from build123d import *

# Parameters (mm, degrees)
SKETCH_1_R          = 1.7
EXTRUDE_1_DEPTH     = 39
FILLET_1_R          = 10
SKETCH_3_R          = 1.7
EXTRUDE_2_DEPTH     = 5
EXTRUDE_START       = -3
SKETCH_4_R          = 1.7
EXTRUDE_3_DEPTH     = 3
CUT_EXTRUDE_2_DEPTH = 5
SKETCH_6_R          = 1.7
EXTRUDE_4_DEPTH     = 3
SKETCH_7_R          = 1.7
EXTRUDE_5_DEPTH     = 5
SKETCH_8_R          = 3
SKETCH_8_R_2        = 1.7
EXTRUDE_6_DEPTH     = 39
SKETCH_9_R          = 1.7
CUT_EXTRUDE_3_DEPTH = 100
FILLET_2_R          = 10


with BuildPart() as part:
    # 草图1 → 凸台-拉伸1 (new body)
    with BuildSketch(Plane(origin=(0, 0, 0), x_dir=(1, 0, 0), z_dir=(0, 1, 0))):
        with BuildLine():
            Line((-14.277701198, -3), (35.505461262, -3))
            ThreePointArc((35.505461262, -3), (36.773316047, -2.718923361), (37.803594591, -1.928362829))
            Line((37.803594591, -1.928362829), (63.497014217, 28.691862316))
            Line((63.497014217, 28.691862316), (61.198880888, 30.620225145))
            Line((61.198880888, 30.620225145), (37.433824091, 2.298133329))
            ThreePointArc((37.433824091, 2.298133329), (34.237606477, 2.718923361), (32.505461262, 0))
            Line((32.505461262, 0), (-11.277701198, 0))
            ThreePointArc((-11.277701198, 0), (-16.399021541, 2.121320344), (-14.277701198, -3))
        make_face()
        with Locations(Location((-14.277701198, 0, 0), (0, 0, 270))):
            Circle(SKETCH_1_R, mode=Mode.SUBTRACT)
        with Locations(Location((35.505461262, 0, 0), (0, 0, 270))):
            Circle(SKETCH_1_R, mode=Mode.SUBTRACT)
    extrude(amount=EXTRUDE_1_DEPTH)

    # 圆角1
    fillet_1_edges = [part.edges().sort_by_distance(p)[0] for p in [
        (37.433824091, 19.5, -2.298133329),
        (-11.277701198, 19.5, 0),
        (32.505461262, 19.5, 0),
    ]]
    fillet(fillet_1_edges, radius=FILLET_1_R)

    # 草图3 → 凸台-拉伸2 (add)
    with BuildSketch(Plane(origin=(0, 0, 0), x_dir=(1, 0, 0), z_dir=(0, 1, 0))):
        with BuildLine():
            Line((-14.277701198, 3), (35.505461262, 3))
            ThreePointArc((35.505461262, 3), (38.505461262, 0), (35.505461262, -3))
            Line((35.505461262, -3), (-14.277701198, -3))
            ThreePointArc((-14.277701198, -3), (-17.277701198, 0), (-14.277701198, 3))
        make_face()
        with Locations(Location((35.505461262, 0, 0), (0, 0, 270))):
            Circle(SKETCH_3_R, mode=Mode.SUBTRACT)
    extrude(amount=EXTRUDE_2_DEPTH)

    # 草图4 → 凸台-拉伸3 (add)
    with BuildSketch(Plane(origin=(0, 39, 0), x_dir=(1, 0, 0), z_dir=(0, 1, 0)).offset(EXTRUDE_START)):
        with BuildLine():
            Line((-14.277701198, 3), (35.505461262, 3))
            ThreePointArc((35.505461262, 3), (38.505461262, 0), (35.505461262, -3))
            Line((35.505461262, -3), (-14.277701198, -3))
            ThreePointArc((-14.277701198, -3), (-17.277701198, 0), (-14.277701198, 3))
        make_face()
        with Locations(Location((-14.277701198, 0, 0), (0, 0, 270))):
            Circle(SKETCH_4_R, mode=Mode.SUBTRACT)
        with Locations(Location((35.505461262, 0, 0), (0, 0, 270))):
            Circle(SKETCH_4_R, mode=Mode.SUBTRACT)
    extrude(amount=EXTRUDE_3_DEPTH)

    # 草图5 → 切除-拉伸2 (cut)
    with BuildSketch(Plane.XY.offset(3)):
        with BuildLine():
            Line((-2.386119968, 30.5), (23.613880032, 30.5))
            ThreePointArc((23.613880032, 30.5), (26.613880032, 27.5), (23.613880032, 24.5))
            Line((23.613880032, 24.5), (-2.386119968, 24.5))
            ThreePointArc((-2.386119968, 24.5), (-5.386119968, 27.5), (-2.386119968, 30.5))
        make_face()
        with BuildLine():
            Line((-2.386119968, 8.5), (23.613880032, 8.5))
            ThreePointArc((23.613880032, 8.5), (26.613880032, 11.5), (23.613880032, 14.5))
            Line((23.613880032, 14.5), (-2.386119968, 14.5))
            ThreePointArc((-2.386119968, 14.5), (-5.386119968, 11.5), (-2.386119968, 8.5))
        make_face()
    extrude(amount=-CUT_EXTRUDE_2_DEPTH, mode=Mode.SUBTRACT)

    # 草图6 → 凸台-拉伸4 (add)
    with BuildSketch(Plane(origin=(0, 39, 0), x_dir=(1, 0, 0), z_dir=(0, 1, 0)).offset(EXTRUDE_START)):
        with BuildLine():
            Line((33.207327933, 1.928362829), (58.890388489, 32.536242516))
            ThreePointArc((58.890388489, 32.536242516), (63.116884647, 32.906013016), (63.486655148, 28.679516858))
            Line((63.486655148, 28.679516858), (37.803594591, -1.928362829))
            ThreePointArc((37.803594591, -1.928362829), (33.577098433, -2.298133329), (33.207327933, 1.928362829))
        make_face()
        with Locations(Location((35.505461262, 0, 0), (0, 0, 270))):
            Circle(SKETCH_6_R, mode=Mode.SUBTRACT)
        with Locations((61.188521818, 30.607879687)):
            Circle(SKETCH_6_R, mode=Mode.SUBTRACT)
    extrude(amount=EXTRUDE_4_DEPTH)

    # 草图7 → 凸台-拉伸5 (add)
    with BuildSketch(Plane(origin=(0, 0, 0), x_dir=(1, 0, 0), z_dir=(0, 1, 0))):
        with BuildLine():
            Line((33.207327933, 1.928362829), (58.890388489, 32.536242516))
            ThreePointArc((58.890388489, 32.536242516), (63.116884647, 32.906013016), (63.486655148, 28.679516858))
            Line((63.486655148, 28.679516858), (37.803594591, -1.928362829))
            ThreePointArc((37.803594591, -1.928362829), (33.577098433, -2.298133329), (33.207327933, 1.928362829))
        make_face()
        with Locations(Location((35.505461262, 0, 0), (0, 0, 270))):
            Circle(SKETCH_7_R, mode=Mode.SUBTRACT)
        with Locations((61.188521818, 30.607879687)):
            Circle(SKETCH_7_R, mode=Mode.SUBTRACT)
    extrude(amount=EXTRUDE_5_DEPTH)

    # 草图8 → 凸台-拉伸6 (add)
    with BuildSketch(Plane(origin=(0, 0, 0), x_dir=(1, 0, 0), z_dir=(0, 1, 0))):
        with Locations((61.188521818, 30.607879687)):
            Circle(SKETCH_8_R)
        with Locations((61.188521818, 30.607879687)):
            Circle(SKETCH_8_R_2, mode=Mode.SUBTRACT)
    extrude(amount=EXTRUDE_6_DEPTH)

    # 草图9 → 切除-拉伸3 (cut)
    with BuildSketch(Plane(origin=(0, 0, 0), x_dir=(1, 0, 0), z_dir=(0, 1, 0))):
        with Locations(Location((61.188521818, 30.607879687, 0), (0, 0, 270))):
            Circle(SKETCH_9_R)
    extrude(amount=CUT_EXTRUDE_3_DEPTH, mode=Mode.SUBTRACT)

    # 圆角2
    fillet_2_edges = [part.edges().sort_by_distance(p)[0] for p in [
        (34.106538287, 37.5, -3),
        (34.106538287, 2.5, -3),
    ]]
    fillet(fillet_2_edges, radius=FILLET_2_R)


solid = part.part
Work out the finished part from the listing and answer in its coordinate system (mm). A direction names the side the tool comes from. Give positions to 0.01 mm unless a question says otherwise; leave off trailing zeros. Order: outer loops, then holes, each group sorted by start corner. A loop starts at its lowest first (then second) coordinate and runs counter-clockwise, first axis right, second up. Notation, with made-up numbers: (43, 81) -> (47, 81) arc R28 cw to (47, 113) -> close; hole circle Ø2 at (-32, 34.25). An arc over 180 degrees is marked (long way). One line per item, written item: value.
Item 1: Find section A-A, the plane y = 11.5. State how many separate pieces and enclosed holes the cut face has, plus the area to 3 significant figures.
Answer sheet:
separate pieces: 2
enclosed holes: 3
area: 211 mm²
Item 2: Find section B-B, the plane x = 21. Give the vertices of the cut face in (y, z).
Answer sheet:
outline: (0, -3) -> (5, -3) -> (5, 0) -> (8.5, 0) -> (8.5, 3) -> (0, 3) -> close; (14.5, 0) -> (24.5, 0) -> (24.5, 3) -> (14.5, 3) -> close; (30.5, 0) -> (36, 0) -> (36, -3) -> (39, -3) -> (39, 3) -> (30.5, 3) -> close
Item 3: Determine the mould class of faces 5 (the cylindrical face through (33.72, 2.54, -3.96)), 6 (the cylindrical face through (36.757, 19.227, 2.727)), 7 (the cylindrical face through (26.613, 27.566, 1.521)) for opening direction X: released by +X, released by -X, zero draft, split by the parting line, or undercut.
Answer sheet:
face 5: released by -X
face 6: released by +X
face 7: undercut
Item 4: Flat-ended cylindrical pins translate along their axes: P1, Ø3, axis at x = -14.28, z = 0, coming from the +Y side; P2, Ø1, axis at x = 40.5, y = 11.5, coming from the +Z side; P3, Ø1, axis at x = 54, y = 5, coming from the +Z side. Find the tip coordinate at first contact, or state that the pin passes through.
Answer sheet:
P1: y = 5
P2: z = -0.69
P3: z = -16.78
Item 5: Find section D-D, the plane x = -9. Give the vertices of the cut face in (y, z), plus the area to 3 significant figures.
Answer sheet:
outline: (0, -3) -> (5, -3) -> (5, -0.47) -> (36, -0.47) -> (36, -3) -> (39, -3) -> (39, 3) -> (0, 3) -> close
area: 156 mm²
Item 6: Straight lines are drawn through the part: probe 1 along Y at (x, z) = (1, 1.5); probe 2 along Y at (x, z) = (56.5, -29.5); probe 3 along Z at (x, y) = (61, 5). For each, find the intervals that lie inside material, in ascending order.
Answer sheet:
probe 1: 0 to 8.5, 14.5 to 24.5, 30.5 to 39
probe 2: 0 to 5, 36 to 39
probe 3: -33.6 to -32.3, -28.92 to -25.72
Item 7: A tool of negligible diameter and unlimited length cuts with its end or side. For faces 1 (the cylindrical face through (-12.59, 21.76, -0.22)), 2 (the flat face through (11, 24, 0)), 3 (the flat face through (47.84, 37.48, -19.37)), 4 (the flat face through (11, 14.5, 2)), from which of +Z, -Z, +X, -X, +Y, -Y can it reach the whole face along a straight path? Write none if from no direction.
Answer sheet:
face 1: +Y
face 2: -Z
face 3: -Z, -X, +Y, -Y
face 4: +Z, -Z
